Autodesk Inventor part; units mm, degrees
ref_plane "YZ Plane" through (0, 0, 0) normal (1, 0, 0) x (0, 1, 0)
ref_plane "XZ Plane" through (0, 0, 0) normal (0, 1, 0) x (-1, 0, 0)
ref_plane "XY Plane" through (0, 0, 0) normal (0, 0, 1) x (1, 0, 0)
sketch "Boceto1" plane through (0, 0, 0) normal (0, 0, 1) x (1, 0, 0)
  circle A0 centre (0, 0) radius 9.525
  circle A1 centre (0, 0) radius 225
  arc A2 (26.9272, -13.2259) -> (26.9272, 13.2259) centre (0, 0) ccw
  arc A3 (174.2011, -98.2546) -> (174.2011, 98.2546) centre (0, 0) ccw
  line L0 (26.9272, 13.2259) -> (174.2011, 98.2546)
  line L1 (26.9272, -13.2259) -> (174.2011, -98.2546)
  line L2 (13.2259, -26.9272) -> (98.2546, -174.2011)
  arc A4 (-98.2546, -174.2011) -> (98.2546, -174.2011) centre (0, 0) ccw
  line L3 (-13.2259, -26.9272) -> (-98.2546, -174.2011)
  arc A5 (-13.2259, -26.9272) -> (13.2259, -26.9272) centre (0, 0) ccw
  line L4 (-26.9272, -13.2259) -> (-174.2011, -98.2546)
  arc A6 (-174.2011, 98.2546) -> (-174.2011, -98.2546) centre (0, 0) ccw
  line L5 (-26.9272, 13.2259) -> (-174.2011, 98.2546)
  arc A7 (-26.9272, 13.2259) -> (-26.9272, -13.2259) centre (0, 0) ccw
  line L6 (-13.2259, 26.9272) -> (-98.2546, 174.2011)
  arc A8 (98.2546, 174.2011) -> (-98.2546, 174.2011) centre (0, 0) ccw
  line L7 (13.2259, 26.9272) -> (98.2546, 174.2011)
  arc A9 (13.2259, 26.9272) -> (-13.2259, 26.9272) centre (0, 0) ccw
  dimension "d2" = 450
  dimension "d3" = 60
  dimension "d4" = 400
  dimension "d11" = 360
extrude "Extrusión1" add sketch "Boceto1" along normal blind 45
Source: CAD feature listing. Evaluate the final solid. Frame: model axes, mm. A direction names the side the tool comes from. Round coordinates to 2 decimals unless told otherwise and drop trailing zeros. Order: outer loops, then holes, each group sorted by start corner. A loop starts at its lowest first (then second) coordinate and runs counter-clockwise, first axis right, second up. Notation, with made-up numbers: (18, -19) -> (69, -19) arc R17 ccw to (69, 9) -> close; hole circle Ø8 at (-17.75, -31.5). An arc over 180 degrees is marked (long way). One line per item, written item: value. Start each with the question number.
Q1. Section query B-B (z = 20). Return the cut outline in (x, y) (3 decimals).
Q2. Pin query (flat end, axial travel): pin 1 (5 mm diameter, centred on x = -24, z = 25.5, fed in from -Y); pin 2 (6 mm diameter, centred on x = -13.5, z = 15, fed in from +Y); pin 3 (1 mm diameter, centred on y = 150.5, z = 26, fed in from +X). Return the tip coordinate at first contact, or that it passes through.
Q3. Draft query along X for faces 3 (the flat face through (47, -47, 0)), 4 (the cylindrical face through (30, 0, 22)), 5 (the cylindrical face through (-224.782, -9.893, 22.185)), 6 (the flat face through (99.533, 55.145, 22.185)). Return one class per face: pulls with the +X half, pulls with the -X half, needs draft (parallel to the pull), parting line crosses it, or undercut.
Q4. Section query D-D (y = -136.5). Return the cut outline in (x, z), plus the area to 3 significant figures.
Q5. Material intervals for probe 1 along Y at (x, z) = (0, 15) (3 decimals); probe 2 along X at (y, z) = (-59, 18); probe 3 along X at (y, z) = (69, 42), sorted ascending.
Q6. Section query A-A (x = 0). Return the cut outline in (y, z) (3 decimals).
Q7. Access query for faces 1 (the flat face through (47, -47, 45)), 2 (the cylindrical face through (-30, 0, 22)). Directions: +Z, -Z, +X, -X, +Y, -Y. A direction counts if a zero-diameter tool reaches every point of the face in a straight line with its end or side. Return the directions, or none.
Findings below:
1. outline: circle Ø450 at (0, 0); hole (-174.201, -98.255) -> (-26.927, -13.226) arc R30 cw to (-26.927, 13.226) -> (-174.201, 98.255) arc R200 ccw to start; hole (-98.255, -174.201) arc R200 ccw to (98.255, -174.201) -> (13.226, -26.927) arc R30 cw to (-13.226, -26.927) -> close; hole (-98.255, 174.201) -> (-13.226, 26.927) arc R30 cw to (13.226, 26.927) -> (98.255, 174.201) arc R200 ccw to start; hole circle Ø19.05 at (0, 0); hole (26.927, -13.226) -> (174.201, -98.255) arc R200 ccw to (174.201, 98.255) -> (26.927, 13.226) arc R30 cw to start
2. pin 1: y = -223.97
2. pin 2: y = 224.75
2. pin 3: x = 167.71
3. face 3: needs draft
3. face 4: undercut
3. face 5: parting line crosses it
3. face 6: undercut
4. outline: (-178.87, 0) -> (-76.49, 0) -> (-76.49, 45) -> (-178.87, 45) -> close; (76.49, 0) -> (178.87, 0) -> (178.87, 45) -> (76.49, 45) -> close
4. area: 9,210 mm²
5. probe 1: -225 to -200, -30 to -9.525, 9.525 to 30, 200 to 225
5. probe 2: -217.13 to -191.1, -106.21 to -31.74, 31.74 to 106.21, 191.1 to 217.13
5. probe 3: -214.16 to -187.72, -123.53 to -37.52, 37.52 to 123.53, 187.72 to 214.16
6. outline: (-225, 0) -> (-200, 0) -> (-200, 45) -> (-225, 45) -> close; (-30, 0) -> (-9.525, 0) -> (-9.525, 45) -> (-30, 45) -> close; (9.525, 0) -> (30, 0) -> (30, 45) -> (9.525, 45) -> close; (200, 0) -> (225, 0) -> (225, 45) -> (200, 45) -> close
7. face 1: +Z, +X, -X, +Y, -Y
7. face 2: +Z, -Z
